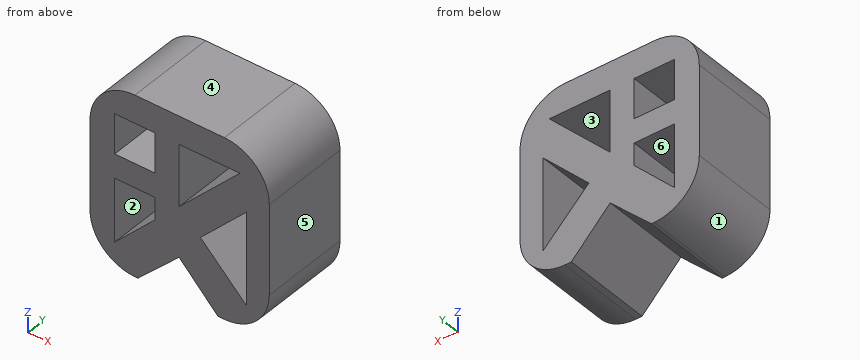
```python
from build123d import *

# Parameters (mm, degrees)
F2_DEPTH = 12.7
F3_DEPTH = 25.4
F4_W     = 7.152606
F4_H     = 3.387249
F5_DEPTH = 12.7
F7_DEPTH = 254


with BuildPart() as f2:
    # F0 (on Front) → F2 (new body)
    with BuildSketch(Plane.XZ):
        with BuildLine():
            Line((-34.402621, 38.858883), (-47.026384, 38.858883))
            ThreePointArc((-47.026384, 38.858883), (-51.516512, 36.999011), (-53.376384, 32.508883))
            Line((-53.376384, 32.508883), (-53.376384, 19.885116))
            ThreePointArc((-53.376384, 19.885116), (-51.516512, 15.394988), (-47.026384, 13.535116))
            Line((-47.026384, 13.535116), (-34.402621, 13.535116))
            ThreePointArc((-34.402621, 13.535116), (-29.912493, 15.394988), (-28.052621, 19.885116))
            Line((-28.052621, 19.885116), (-28.052621, 32.508883))
            ThreePointArc((-28.052621, 32.508883), (-29.912493, 36.999011), (-34.402621, 38.858883))
        make_face()
    extrude(amount=F2_DEPTH)

    # F1 (on Front) → F3 (cut, symmetric)
    with BuildSketch(Plane.XZ):
        Polygon((-32.199131, 34.929331), (-49.883451, 34.929331), (-49.883451, 17.02805), align=None)
        Polygon((-31.301971, 16.947381), (-31.301971, 29.916352), (-37.785975, 23.3528), align=None)
    extrude(amount=F3_DEPTH, both=True, mode=Mode.SUBTRACT)

    # F4 (on Front) → F5 (join)
    with BuildSketch(Plane.XZ):
        Polygon((-44.176444, 25.931474), (-44.176444, 21.922855), (-40.789195, 21.922855), (-40.789195, 36.714591), (-44.176444, 36.714591), (-44.176444, 29.318723), align=None)
        with Locations((-47.752747, 27.625099)):
            Rectangle(F4_W, F4_H)
    extrude(amount=F5_DEPTH)

    # F6 (on face) → F7 (cut)
    with BuildSketch(Plane(origin=(0, 0, 0), x_dir=(-1, 0, 0), z_dir=(0, 1, 0))):
        Polygon((35.308003, 13.535116), (46.605372, 13.535116), (40.789195, 19.181317), align=None)
        Polygon((33.403759, 11.573545), (47.081295, 13.073102), (46.605372, 13.535116), (35.308003, 13.535116), align=None)
    extrude(amount=-F7_DEPTH, mode=Mode.SUBTRACT)


solid = f2.part
```
Part model, mm, in its own coordinate system. Face numbers are marked on the shaded views. A direction names the side the tool comes from. Round coordinates to 2 decimals unless told otherwise and drop trailing zeros. Write each loop counter-clockwise with the first axis right and the second up, starting at its lowest first coordinate (ties: lowest second). Pieces come first, ordered by that corner, then holes. Notation, with made-up numbers: M 43.5,-39 L 60.5,-39 A23 cw 60.5,-8 Z; hole C 46.25,86.5 d9. An arc over 180 degrees is marked long. One line per question, with ' | ' between items.
(1) Pin check, flat tips, straight feed: pin 1 (6 mm diameter, centred on x = -48, z = 33.5, fed in from -Y); pin 2 (4 mm diameter, centred on x = -50, y = -11.5, fed in from -Z); pin 3 (1.5 mm diameter, centred on x = -44, y = -11, fed in from -Z). Stop position of each tip, or through.
Answer key:
pin 1: stops at y = -12.7 | pin 2: stops at z = 13.61 | pin 3: stops at z = 15.34
(2) Two-plate mould, pull along Z, no slides. Class the marked faces 3, 4, 5 and 6: released by +Z, released by -Z, zero draft, split by the parting line, or undercut.
Answer key:
face 3: undercut | face 4: released by +Z | face 5: zero draft | face 6: undercut
(3) Saw through at B-B on x = -36.75. Write the cut outline in (y, z), then the cut area to 3 significant figures.
Answer key:
outline: M -12.7,15.02 L 0,15.02 L 0,22.33 L -12.7,22.33 Z; M -12.7,24.4 L 0,24.4 L 0,30.32 L -12.7,30.32 Z; M -12.7,34.93 L 0,34.93 L 0,38.86 L -12.7,38.86 Z | area: 218 mm^2
(4) Saw through at A-A on z = 21.5. Write the cut outline in (x, y), then the cut area to 3 significant figures.
Answer key:
outline: M -53.38,-12.7 L -49.88,-12.7 L -49.88,0 L -53.38,0 Z; M -45.47,-12.7 L -35.91,-12.7 L -35.91,0 L -45.47,0 Z; M -31.3,-12.7 L -28.05,-12.7 L -28.05,0 L -31.3,0 Z | area: 207 mm^2
(5) Probe line 1 along X through (y, z) = (-4.5, 33.5); line 2 along Z through (x, y) = (-36, -8.75); line 3 along X through (y, z) = (-3, 27.5). List the from-to ranges inside material, lowest first.
Answer key:
line 1: x = -53.3 to -49.88, -44.18 to -40.79, -33.61 to -28.13 | line 2: z = 14.25 to 21.59, 25.16 to 31.08, 34.93 to 38.86 | line 3: x = -53.38 to -40.79, -39.54 to -33.69, -31.3 to -28.05
(6) 3-axis set-ups, long thin cutter, end or side, ignore diameter. For the marked faces 1 and 2: which of +Z, -Z, +X, -X, +Y, -Y reach the whole face in a straight line?
Answer key:
face 1: -Z, -X, +Y, -Y | face 2: +Y, -Y
(7) Saw through at D-D on z = 15.25. Write the cut outline in (x, y).
Answer key:
outline: M -51.37,-12.7 L -44.84,-12.7 L -44.84,0 L -51.37,0 Z; M -36.97,-12.7 L -30.06,-12.7 L -30.06,0 L -36.97,0 Z
(8) Saw through at C-C on y = -5.5. Write the cut outline in (x, z).
Answer key:
outline: M -53.38,19.89 A6.35 ccw -47.03,13.54 L -46.61,13.54 L -40.79,19.18 L -35.31,13.54 L -34.4,13.54 A6.35 ccw -28.05,19.89 L -28.05,32.51 A6.35 ccw -34.4,38.86 L -47.03,38.86 A6.35 ccw -53.38,32.51 Z; hole M -49.88,17.03 L -44.18,22.81 L -44.18,25.93 L -49.88,25.93 Z; hole M -49.88,29.32 L -44.18,29.32 L -44.18,34.93 L -49.88,34.93 Z; hole M -40.79,26.23 L -32.2,34.93 L -40.79,34.93 Z; hole M -37.79,23.35 L -31.3,16.95 L -31.3,29.92 Z
